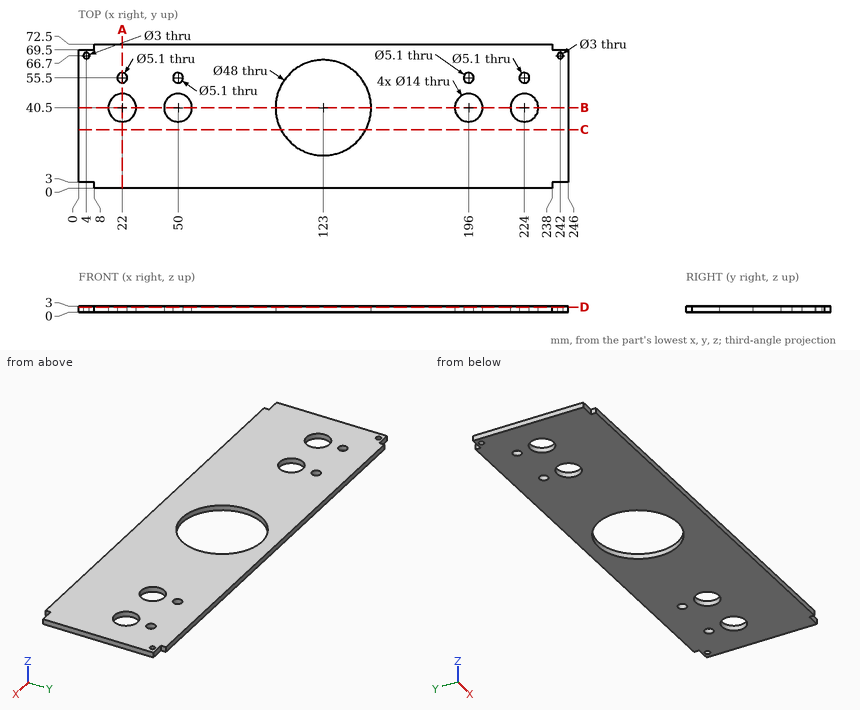
Design review of the part shown in the three views and the two pictorial views. Dimensions are in mm from the part's minimum x, y and z. Round coordinates to 2 decimals unless told otherwise and drop trailing zeros. Loops run counter-clockwise (first coordinate to the right, second up) from the corner with the lowest first, then second, coordinate; pieces in that order, holes last. Notation, with made-up numbers: M 7,83.5 L 63,83.5 A29 ccw 63,104.5 Z; hole C -30,78 d1. An arc over 180 degrees is marked long. Answer as a JSON object with one key per item and string values.
Item 1: For line 1 along X through (y, z) = (66.7, 1.25); line 2 along Y through (x, z) = (224, 1.7); line 3 along Y through (x, z) = (123, 1), list the stretches that pass through material, from the lowest coordinate up.
Check sheet entries:
{"line 1": "0 to 2.5, 5.5 to 240.5, 243.5 to 246", "line 2": "0 to 33.5, 47.5 to 52.95, 58.05 to 72.5", "line 3": "0 to 16.5, 64.5 to 72.5"}
Item 2: Clearance check with flat-ended pins moving along their axes: P1, Ø4.5, axis at x = 22, y = 55.5, coming from the +Z side; P2, Ø1.5, axis at x = 243.5, z = 2, coming from the +Y side; P3, Ø0.9, axis at x = 5.5, z = 1.5, coming from the -Y side. State where each tip first meets the part, or that it passes through.
Check sheet entries:
{"P1": "through", "P2": "y = 69.5", "P3": "y = 3"}
Item 3: We need section B-B, the plane y = 40.5. State the section outline as (x, z) points, and give its area (3 significant figures).
Check sheet entries:
{"outline": "M 0,0 L 15,0 L 15,3 L 0,3 Z; M 29,0 L 43,0 L 43,3 L 29,3 Z; M 57,0 L 99,0 L 99,3 L 57,3 Z; M 147,0 L 189,0 L 189,3 L 147,3 Z; M 203,0 L 217,0 L 217,3 L 203,3 Z; M 231,0 L 246,0 L 246,3 L 231,3 Z", "area": "426 mm2"}
Item 4: We need section D-D, the plane z = 2.55. State how many separate pieces and enclosed holes the cut face has, and give its area (3 significant figures).
Check sheet entries:
{"separate pieces": "1", "enclosed holes": "11", "area": "15,200 mm2"}
Item 5: We need section C-C, the plane y = 29.5. State the section outline as (x, z) points.
Check sheet entries:
{"outline": "M 0,0 L 101.67,0 L 101.67,3 L 0,3 Z; M 144.33,0 L 246,0 L 246,3 L 144.33,3 Z"}
Item 6: We need section A-A, the plane x = 22. State the section outline as (y, z) points.
Check sheet entries:
{"outline": "M 0,0 L 33.5,0 L 33.5,3 L 0,3 Z; M 47.5,0 L 52.95,0 L 52.95,3 L 47.5,3 Z; M 58.05,0 L 72.5,0 L 72.5,3 L 58.05,3 Z"}
